Read the model definition and answer for the solid it produces. Units are mm, in the model's axes. Face numbers are marked on the shaded views. A direction names the side the tool comes from. Round coordinates to 2 decimals unless told otherwise and drop trailing zeros. Order: outer loops, then holes, each group sorted by start corner. A loop starts at its lowest first (then second) coordinate and runs counter-clockwise, first axis right, second up. Notation, with made-up numbers: (-34.75, 54) -> (-7.75, 54) arc R10 ccw to (-7.75, 68) -> close; hole circle Ø5 at (-33, -34.5). An arc over 180 degrees is marked (long way). One line per item, written item: value. Start each with the question number.
1. Section C-C (x = -66) is taken. Give the vertices of the cut face in (y, z), then the cut area to 3 significant figures.
2. Consider line 1 (X direction, y = 1.75, z = 15.5); line 2 (X direction, y = 0.75, z = 12); line 3 (Y direction, x = -10, z = 6). Determine where each line is inside the solid, lowest interval first.
3. For the marked faces 5, 6 and 7, determine the directions among +Z, -Z, +X, -X, +Y, -Y from which every point of the face is accessible in a straight line to the end or side of a thin tool.
4. Flat-ended cylindrical pins translate along their axes: pin 1 Ø4 at (x, y) = (7, -8.5) entering from -Z; pin 2 Ø11 at (x, y) = (-64, 2.5) entering from +Z; pin 3 Ø5.5 at (x, y) = (-19, -8.5) entering from +Z; pin 4 Ø1.8 at (y, z) = (3, 31) entering from -X. Find the tip coordinate at first contact, or state that the pin passes through.
5. Section B-B (z = -2.5) is taken. Give the vertices of the cut face in (x, y).
6. Section A-A (x = 19) is taken. Give the vertices of the cut face in (y, z), then the cut area to 4 significant figures.
7. Section D-D (x = -32) is taken. Give the vertices of the cut face in (y, z), then the cut area to 3 significant figures.
8. The mould has two halves that part along Z. Classify the marked faces 1, 2, 3 and 4: released by +Z, released by -Z, zero draft, split by the parting line, or undercut.
from build123d import *

# Parameters (mm, degrees)
SKETCH_1_W                 = 50
SKETCH_1_H                 = 22
EXTRUDE_1_DEPTH            = 35
SKETCH_2_R                 = 1.27968475
SKETCH_2_R_2               = 1.164740644
CUT_EXTRUDE_1_DEPTH        = 10
HOLE_WIZARD_1_2_13_1_D     = 10.71626
HOLE_WIZARD_1_2_13_1_DEPTH = 31.26
HOLE_WIZARD_1_2_13_1_TIP   = 3.219489309
CUT_EXTRUDE_2_REACH        = 46.396
SKETCH_5_R                 = 1.75
SKETCH_6_W                 = 35
SKETCH_6_H                 = 22
EXTRUDE_3_DEPTH            = 7
SKETCH_7_W                 = 34.8
SKETCH_7_H                 = 21.8
EXTRUDE_4_DEPTH            = 25
SKETCH_8_W                 = 60
SKETCH_8_H                 = 21.8
EXTRUDE_5_DEPTH            = 30
SKETCH_9_R                 = 9.5
EXTRUDE_6_DEPTH            = 25
SKETCH_10_R                = 9.084139512
EXTRUDE_7_DEPTH            = 8
FILLET_1_R                 = 2


with BuildPart() as part:
    # 草图1 → 凸台-拉伸1 (new body)
    with BuildSketch(Plane.XY):
        Rectangle(SKETCH_1_W, SKETCH_1_H)
    extrude(amount=EXTRUDE_1_DEPTH)

    # 草图2 → 切除-拉伸1 (cut)
    with BuildSketch(Plane(origin=(0, 0, 0), x_dir=(-1, 0, 0), z_dir=(0, 0, -1))):
        with Locations((-10, -1)):
            Circle(SKETCH_2_R)
        with Locations((10, 1)):
            Circle(SKETCH_2_R_2)
    extrude(amount=-CUT_EXTRUDE_1_DEPTH, mode=Mode.SUBTRACT)

    # 1/2-13 螺纹孔1
    with Locations(Plane(origin=(0, 0, 0), x_dir=(-1, 0, 0), z_dir=(0, 0, -1))):
        with Locations((10, 1), (-10, -1)):
            Hole(HOLE_WIZARD_1_2_13_1_D / 2, depth=HOLE_WIZARD_1_2_13_1_DEPTH)
            with Locations((0, 0, -(HOLE_WIZARD_1_2_13_1_DEPTH + HOLE_WIZARD_1_2_13_1_TIP / 2))):  # 118° drill point
                Cone(0, HOLE_WIZARD_1_2_13_1_D / 2, HOLE_WIZARD_1_2_13_1_TIP, mode=Mode.SUBTRACT)

    # 草图5 → 切除-拉伸2 (cut, up to next)
    with BuildSketch(Plane(origin=(0, 0, 0), x_dir=(-1, 0, 0), z_dir=(0, 0, -1)), mode=Mode.PRIVATE) as cut_extrude_2_sk1:
        with Locations((-19, 8.5)):
            Circle(SKETCH_5_R)
    cut_extrude_2_tool1 = extrude(cut_extrude_2_sk1.sketch, amount=-CUT_EXTRUDE_2_REACH, mode=Mode.PRIVATE) & part.part
    # 草图5 → 切除-拉伸2 (cut, up to next)
    with BuildSketch(Plane(origin=(0, 0, 0), x_dir=(-1, 0, 0), z_dir=(0, 0, -1)), mode=Mode.PRIVATE) as cut_extrude_2_sk2:
        with Locations((19, -8.5)):
            Circle(SKETCH_5_R)
    cut_extrude_2_tool2 = extrude(cut_extrude_2_sk2.sketch, amount=-CUT_EXTRUDE_2_REACH, mode=Mode.PRIVATE) & part.part
    add(cut_extrude_2_tool1.solids().sort_by_distance((19, 8.5, 0))[0], mode=Mode.SUBTRACT)
    add(cut_extrude_2_tool2.solids().sort_by_distance((-19, -8.5, 0))[0], mode=Mode.SUBTRACT)

    # 草图6 → 凸台-拉伸3 (add)
    with BuildSketch(Plane(origin=(25, 0, 0), x_dir=(0, 0, -1), z_dir=(1, 0, 0))):
        with Locations((-17.5, 0)):
            Rectangle(SKETCH_6_W, SKETCH_6_H)
    extrude(amount=EXTRUDE_3_DEPTH)

    # 草图7 → 凸台-拉伸4 (add)
    with BuildSketch(Plane.ZY.offset(25)):
        with Locations((17.5, 0)):
            Rectangle(SKETCH_7_W, SKETCH_7_H)
    extrude(amount=EXTRUDE_4_DEPTH)

    # 草图8 → 凸台-拉伸5 (add)
    with BuildSketch(Plane.ZY.offset(50)):
        with Locations((-1.1, 0)):
            Rectangle(SKETCH_8_W, SKETCH_8_H)
    extrude(amount=EXTRUDE_5_DEPTH)

    # 草图9 → 凸台-拉伸6 (add)
    with BuildSketch(Plane(origin=(-50, 0, 0), x_dir=(0, 0, -1), z_dir=(1, 0, 0))):
        with Locations(Location((21.1, 0, 0), (0, 0, 180))):
            Circle(SKETCH_9_R)
    extrude(amount=EXTRUDE_6_DEPTH)

    # 草图10 → 凸台-拉伸7 (add)
    with BuildSketch(Plane.ZY.offset(80)):
        with Locations((16.280298675, 0)):
            Circle(SKETCH_10_R)
    extrude(amount=EXTRUDE_7_DEPTH)

    # 圆角1
    fillet_1_edges = [part.edges().sort_by_distance(p)[0] for p in [
        (-88, 0, 7.196159162),
    ]]
    fillet(fillet_1_edges, radius=FILLET_1_R)


solid = part.part
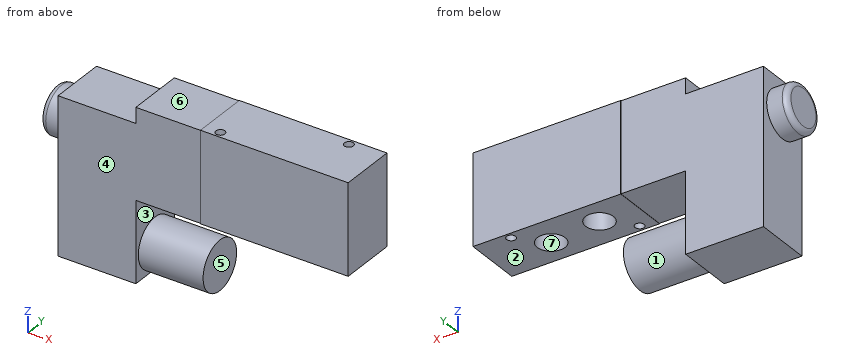
Answer:
1. outline: (-10.9, -31.1) -> (10.9, -31.1) -> (10.9, 28.9) -> (-10.9, 28.9) -> close
1. area: 1,310 mm^2
2. line 1: -88 to -15.31, -4.69 to 5.4, 14.6 to 32
2. line 2: -88 to -15.35, -4.65 to 4.94, 15.06 to 32
2. line 3: -11 to -4.36, 6.36 to 11
3. face 5: -Z, +X, +Y, -Y
3. face 6: +Z, -X, +Y, -Y
3. face 7: -Z
4. pin 1: z = 0
4. pin 2: z = 28.9
4. pin 3: z = 35
4. pin 4: x = -50
5. outline: (-80, -10.9) -> (-50, -10.9) -> (-50, 10.9) -> (-80, 10.9) -> close
6. outline: (-11, 0) -> (6.75, 0) -> (6.75, 35) -> (-11, 35) -> close; (10.25, 0) -> (11, 0) -> (11, 35) -> (10.25, 35) -> close
6. area: 647.5 mm^2
7. outline: (-10.9, 0.1) -> (10.9, 0.1) -> (10.9, 34.9) -> (-10.9, 34.9) -> close; circle Ø19 at (0, -21.1)
7. area: 1,040 mm^2
8. face 1: undercut
8. face 2: released by -Z
8. face 3: undercut
8. face 4: zero draft
